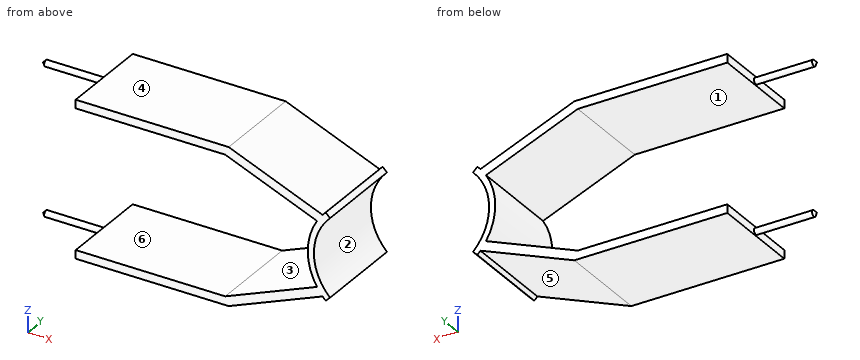
from build123d import *

# Parameters (mm, degrees)
BOSS_EXTRUDE2_DEPTH      = 30
BOSS_EXTRUDE3_START      = -30
BOSS_EXTRUDE3_DEPTH      = 30
BOSS_EXTRUDE4_DEPTH      = 30
SKETCH15_R               = 1
BOSS_EXTRUDE5_DEPTH      = 20
CHAMFER1_SIZE            = 1
CHAMFER1_OF_MIRROR2_SIZE = 1


with BuildPart() as part:
    # Sketch5 → Boss-Extrude2 (new body)
    with BuildSketch(Plane(origin=(0, 0, 0), x_dir=(1, 0, 0), z_dir=(0, 1, 0))):
        with BuildLine():
            Line((-12.727922061, 12.727922061), (-14.142135624, 14.142135624))
            ThreePointArc((-14.142135624, 14.142135624), (-20, 0), (-14.142135624, -14.142135624))
            Line((-14.142135624, -14.142135624), (-12.727922061, -12.727922061))
            ThreePointArc((-12.727922061, -12.727922061), (-18, 0), (-12.727922061, 12.727922061))
        make_face()
    extrude(amount=BOSS_EXTRUDE2_DEPTH)

    # Sketch12 → Boss-Extrude3 (add)
    with BuildSketch(Plane(origin=(0, 30, 0), x_dir=(1, 0, 0), z_dir=(0, 1, 0)).offset(BOSS_EXTRUDE3_START)):
        with BuildLine():
            Line((-16.979679072, 10.568372562), (-46.979679072, 22.693353002))
            Line((-46.979679072, 22.693353002), (-45.855525051, 25.474769501))
            Line((-45.855525051, 25.474769501), (-15.144925587, 13.062588907))
            ThreePointArc((-15.144925587, 13.062588907), (-14.653475488, 13.611600058), (-14.142135624, 14.142135624))
            Line((-14.142135624, 14.142135624), (-12.727922061, 12.727922061))
            ThreePointArc((-12.727922061, 12.727922061), (-18, 0), (-12.727922061, -12.727922061))
            Line((-12.727922061, -12.727922061), (-14.142135624, -14.142135624))
            ThreePointArc((-14.142135624, -14.142135624), (-19.869427299, -2.281635118), (-16.979679072, 10.568372562))
        make_face()
    boss_extrude3 = extrude(amount=BOSS_EXTRUDE3_DEPTH)

    # Sketch14 → Boss-Extrude4 (add)
    with BuildSketch(Plane(origin=(0, 30, 0), x_dir=(1, 0, 0), z_dir=(0, 1, 0))):
        Polygon((-45.855525051, 25.474769501), (-95.855525051, 25.474769501), (-95.855525051, 22.693353002), (-46.979679072, 22.693353002), align=None)
    boss_extrude4 = extrude(amount=-BOSS_EXTRUDE4_DEPTH)

    # Mirror1: Boss-Extrude3, Boss-Extrude4 across plane
    add(boss_extrude3.mirror(Plane(origin=(0, 0, 0), x_dir=(1, 0, 0), z_dir=(0, 0, -1))))
    add(boss_extrude4.mirror(Plane(origin=(0, 0, 0), x_dir=(1, 0, 0), z_dir=(0, 0, -1))))

    # Sketch15 → Boss-Extrude5 (add)
    with BuildSketch(Plane.ZY.offset(95.855525051)):
        with Locations(Location((24.084061252, 15, 0), (0, 0, 180))):
            Circle(SKETCH15_R)
    boss_extrude5 = extrude(amount=BOSS_EXTRUDE5_DEPTH)

    # Chamfer1
    chamfer1_edges = [part.edges().sort_by_distance(p)[0] for p in [
        (-115.855525051, 15, 25.084061252),
    ]]
    chamfer(chamfer1_edges, length=CHAMFER1_SIZE)

    # Mirror2: Boss-Extrude5 across plane
    add(boss_extrude5.mirror(Plane(origin=(0, 0, 0), x_dir=(1, 0, 0), z_dir=(0, 0, -1))))

    # Chamfer1 of Mirror2
    chamfer1_of_mirror2_edges = [part.edges().sort_by_distance(p)[0] for p in [
        (-115.855525051, 15, -25.084061252),
    ]]
    chamfer(chamfer1_of_mirror2_edges, length=CHAMFER1_OF_MIRROR2_SIZE)


solid = part.part
Model file for the job. Use its own axes, mm. Face numbers are marked on the shaded views. A direction names the side the tool comes from. Round coordinates to 2 decimals unless told otherwise and drop trailing zeros. Loops run counter-clockwise (first coordinate to the right, second up) from the corner with the lowest first, then second, coordinate; pieces in that order, holes last.
1. Band-saw the part on B-B, the plane y = 6.5. List the corners of the cut face in (x, z), and give its area (3 significant figures).
Check values:
outline: (-95.86, -25.47) - (-45.86, -25.47) - (-15.14, -13.06) arc R20 ccw to (-14.14, -14.14) - (-12.73, -12.73) arc R18 cw to (-12.73, 12.73) - (-14.14, 14.14) arc R20 ccw to (-15.14, 13.06) - (-45.86, 25.47) - (-95.86, 25.47) - (-95.86, 22.69) - (-46.98, 22.69) - (-16.98, 10.57) arc R20 ccw to (-16.98, -10.57) - (-46.98, -22.69) - (-95.86, -22.69) - close
area: 531 mm2
2. Band-saw the part on C-C, the plane x = -27. List the corners of the cut face in (y, z), and give its area (3 significant figures).
Check values:
outline: (0, -17.85) - (30, -17.85) - (30, -14.62) - (0, -14.62) - close; (0, 14.62) - (30, 14.62) - (30, 17.85) - (0, 17.85) - close
area: 194 mm2
3. Band-saw the part on A-A, the plane x = -107.5. List the corners of the cut face in (y, z), and give its area (3 significant figures).
Check values:
outline: circle Ø2 at (15, -24.08); circle Ø2 at (15, 24.08)
area: 6.28 mm2
4. Wall check: probe 1 along Z at (x, y) = (-71, 12.75); probe 2 along Z at (x, y) = (-27.5, 7.5); probe 3 along X at (y, z) = (22.5, -0.5). Give the ranges that are in metal, low to high.
Check values:
probe 1: z = -25.47 to -22.69, 22.69 to 25.47
probe 2: z = -18.06 to -14.82, 14.82 to 18.06
probe 3: x = -19.99 to -17.99
5. Mould opens along Z. For the marked faces 3, 4, 5 and 6 say: +Z half, -Z half, draft (parallel to the pull), parting line (faces both ways), or undercut.
Check values:
face 3: undercut
face 4: +Z half
face 5: -Z half
face 6: undercut
6. Tool access for the marked faces 1 and 2: list every direction of +Z, -Z, +X, -X, +Y, -Y with a clear straight run to the whole face (end or side of a thin tool).
Check values:
face 1: -X, +Y, -Y
face 2: +X, +Y, -Y
7. Drop flat-ended pins along their axis: P1, Ø1, axis at x = -39.5, y = 26.5, coming from the -Z side; P2, Ø1, axis at y = 25, z = 17, coming from the +X side; P3, Ø8, axis at x = -33.5, y = 23.5, coming from the +Z side. Give the stop position or say it passes through.
Check values:
P1: stops at z = -23.11
P2: stops at x = -23.65
P3: stops at z = 22.1
8. Band-saw the part on D-D, the plane z = 18. List the corners of the cut face in (x, y).
Check values:
outline: (-35.37, 0) - (-27.36, 0) - (-27.36, 30) - (-35.37, 30) - close
